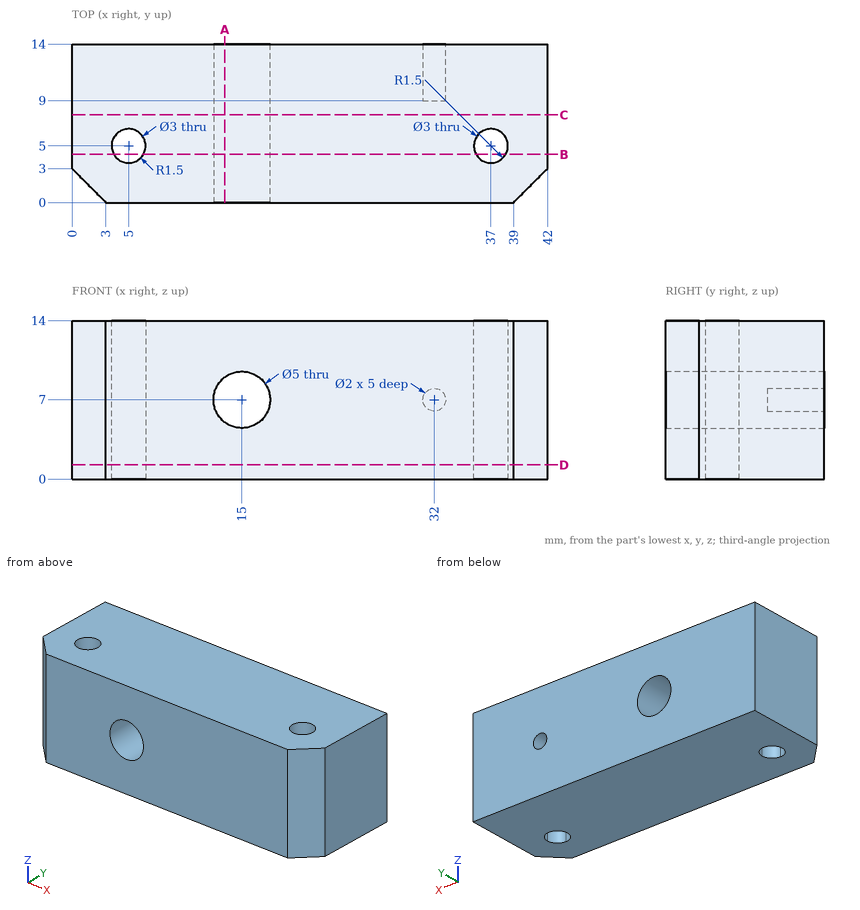
Can you work these out from the drawing? Everything is in mm from the part's minimum corner. Round coordinates to 2 decimals unless told otherwise and drop trailing zeros. Loops run counter-clockwise (first coordinate to the right, second up) from the corner with the lowest first, then second, coordinate; pieces in that order, holes last.
1. If we section it at C-C on y = 7.75: Write out the boundary of the cut face in (x, z).
Answer list:
outline: (0, 0) - (42, 0) - (42, 14) - (0, 14) - close; hole circle Ø5 at (15, 7)
2. If we section it at B-B on y = 4.25: Write out the boundary of the cut face in (x, z).
Answer list:
outline: (0, 0) - (3.7, 0) - (3.7, 14) - (0, 14) - close; (6.3, 0) - (35.7, 0) - (35.7, 14) - (6.3, 14) - close; (38.3, 0) - (42, 0) - (42, 14) - (38.3, 14) - close; hole circle Ø5 at (15, 7)
3. If we section it at A-A on x = 13.5: Write out the boundary of the cut face in (y, z).
Answer list:
outline: (0, 0) - (14, 0) - (14, 5) - (0, 5) - close; (0, 9) - (14, 9) - (14, 14) - (0, 14) - close
4. If I drill on line 1 along X through (y, z) = (5, 9.75); line 2 along X through (y, z) = (5, 7.25); line 3 along X through (y, z) = (4.5, 9.75), over which ranges is the centre line in solid material (lowest first)?
Answer list:
line 1: x = 0 to 3.5, 6.5 to 35.5, 38.5 to 42
line 2: x = 0 to 3.5, 6.5 to 12.51, 17.49 to 35.5, 38.5 to 42
line 3: x = 0 to 3.59, 6.41 to 35.59, 38.41 to 42
5. If we section it at D-D on z = 1.25: Write out the boundary of the cut face in (x, y), plus the area to 3 significant figures.
Answer list:
outline: (0, 3) - (3, 0) - (39, 0) - (42, 3) - (42, 14) - (0, 14) - close; hole circle Ø3 at (5, 5); hole circle Ø3 at (37, 5)
area: 565 mm2
